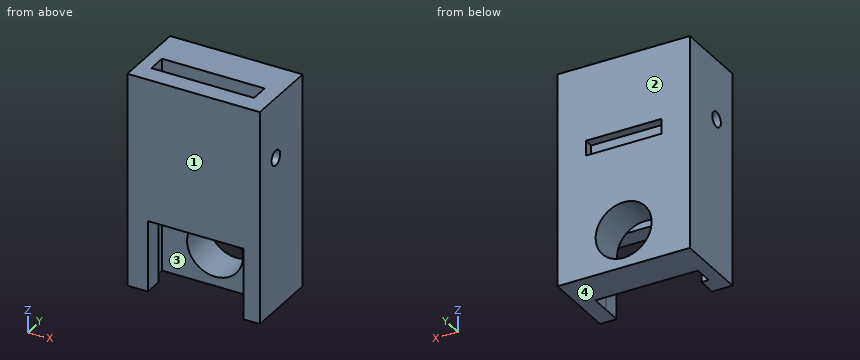
```python
from build123d import *

# Parameters (mm, degrees)
SKETCH1_W           = 71
SKETCH1_H           = 64.24
BOSS_EXTRUDE1_DEPTH = 40
SKETCH2_R           = 4
CUT_EXTRUDE2_DEPTH  = 10
SKETCH5_W           = 71
SKETCH5_H           = 40
BOSS_EXTRUDE2_DEPTH = 50
SKETCH6_R           = 15
CUT_EXTRUDE3_DEPTH  = 98.999716326
SKETCH8_W           = 40.5
SKETCH8_H           = 8
CUT_EXTRUDE5_DEPTH  = 5
CUT_EXTRUDE6_START  = -10
SKETCH9_R           = 4
CUT_EXTRUDE6_DEPTH  = 10
SKETCH10_W          = 55
SKETCH10_H          = 10
CUT_EXTRUDE7_DEPTH  = 127.138921828
SKETCH11_W          = 51.11
SKETCH11_H          = 38
CUT_EXTRUDE8_DEPTH  = 10


with BuildPart() as part:
    # Sketch1 → Boss-Extrude1 (new body)
    with BuildSketch(Plane(origin=(0, 0, 0), x_dir=(1, 0, 0), z_dir=(0, 1, 0))):
        Rectangle(SKETCH1_W, SKETCH1_H)
    extrude(amount=BOSS_EXTRUDE1_DEPTH)

    # Sketch2 → Cut-Extrude2 (cut)
    with BuildSketch(Plane.ZY.offset(35.5)):
        with Locations((-0.12, 15)):
            Circle(SKETCH2_R)
    extrude(amount=-CUT_EXTRUDE2_DEPTH, mode=Mode.SUBTRACT)

    # Sketch5 → Boss-Extrude2 (add)
    with BuildSketch(Plane(origin=(0, 0, -32.12), x_dir=(-1, 0, 0), z_dir=(0, 0, -1))):
        with Locations((0, 20)):
            Rectangle(SKETCH5_W, SKETCH5_H)
    extrude(amount=BOSS_EXTRUDE2_DEPTH)

    # Sketch6 → Cut-Extrude3 (cut, through all)
    with BuildSketch(Plane(origin=(0, 40, 0), x_dir=(1, 0, 0), z_dir=(0, 1, 0))):
        with Locations(Location((0, 62.12, 0), (0, 0, 270))):
            Circle(SKETCH6_R)
    extrude(amount=-CUT_EXTRUDE3_DEPTH, mode=Mode.SUBTRACT)

    # Sketch8 → Cut-Extrude5 (cut)
    with BuildSketch(Plane(origin=(0, 40, 0), x_dir=(1, 0, 0), z_dir=(0, 1, 0))):
        with Locations((0, 12.13)):
            Rectangle(SKETCH8_W, SKETCH8_H)
    extrude(amount=-CUT_EXTRUDE5_DEPTH, mode=Mode.SUBTRACT)

    # Sketch9 → Cut-Extrude6 (cut)
    with BuildSketch(Plane(origin=(35.5, 0, 0), x_dir=(0, 0, -1), z_dir=(1, 0, 0)).offset(CUT_EXTRUDE6_START)):
        with Locations(Location((0.12, 15, 0), (0, 0, 180))):
            Circle(SKETCH9_R)
    extrude(amount=CUT_EXTRUDE6_DEPTH, mode=Mode.SUBTRACT)

    # Sketch10 → Cut-Extrude7 (cut, through all)
    with BuildSketch(Plane.XY.offset(32.12)):
        with Locations((-0.890825636, 15)):
            Rectangle(SKETCH10_W, SKETCH10_H)
    extrude(amount=-CUT_EXTRUDE7_DEPTH, mode=Mode.SUBTRACT)

    # Sketch11 → Cut-Extrude8 (cut)
    with BuildSketch(Plane(origin=(0, 0, 0), x_dir=(-1, 0, 0), z_dir=(0, -1, 0))):
        with Locations((-1.055, 63.12)):
            Rectangle(SKETCH11_W, SKETCH11_H)
    extrude(amount=-CUT_EXTRUDE8_DEPTH, mode=Mode.SUBTRACT)


solid = part.part
```
Work out the finished part from the listing and answer in its coordinate system (mm). Face numbers are marked on the shaded views. Round coordinates to 2 decimals unless told otherwise and drop trailing zeros. Order: outer loops, then holes, each group sorted by start corner. A loop starts at its lowest first (then second) coordinate and runs counter-clockwise, first axis right, second up.
Q1. A cutting plane is placed at C-C, the plane z = -0.12. Determine the outline of the cut face in (x, y).
Solution:
outline: (-35.5, 0) - (35.5, 0) - (35.5, 11) - (26.61, 11) - (26.61, 10) - (-28.39, 10) - (-28.39, 11) - (-35.5, 11) - close; (-35.5, 19) - (-28.39, 19) - (-28.39, 20) - (26.61, 20) - (26.61, 19) - (35.5, 19) - (35.5, 40) - (-35.5, 40) - close
Q2. Given pin 1 Ø8 at (x, y) = (10.5, 5) entering from -Z; pin 2 Ø6.5 at (y, z) = (15, -0.12) entering from +X; pin 3 Ø4 at (x, z) = (9.5, -13.5) entering from +Y; pin 4 Ø1 at (x, z) = (14.5, -65.5) entering from -Y, each flat-ended and moving along its own axis, determine where each tip first touches the part or whether it passes through.
Solution:
pin 1: stops at z = -44.12
pin 2: passes through
pin 3: stops at y = 35
pin 4: stops at y = 20
Q3. Find the intervals of material crossed by line 1 along X through (y, z) = (30.25, -62.12); line 2 along Z through (x, y) = (29.5, 15); line 3 along Y through (x, z) = (33, -0.12), in increasing order.
Solution:
line 1: x = -35.5 to -15, 15 to 35.5
line 2: z = -82.12 to -4.12, 3.88 to 32.12
line 3: y = 0 to 11, 19 to 40
Q4. A cutting plane is placed at A-A, the plane x = 22. Determine the outline of the cut face in (y, z), then the cut area to 3 significant figures.
Solution:
outline: (0, -44.12) - (10, -44.12) - (10, 32.12) - (0, 32.12) - close; (20, -82.12) - (40, -82.12) - (40, 32.12) - (20, 32.12) - close
area: 3,050 mm2
Q5. A cutting plane is placed at D-D, the plane x = 0. Determine the outline of the cut face in (y, z).
Solution:
outline: (0, -44.12) - (10, -44.12) - (10, 32.12) - (0, 32.12) - close; (20, -82.12) - (40, -82.12) - (40, -77.12) - (20, -77.12) - close; (20, -47.12) - (40, -47.12) - (40, -16.13) - (35, -16.13) - (35, -8.13) - (40, -8.13) - (40, 32.12) - (20, 32.12) - close
Q6. A cutting plane is placed at B-B, the plane y = 15. Determine the outline of the cut face in (x, z).
Solution:
outline: (-35.5, -82.12) - (-28.39, -82.12) - (-28.39, -4.12) - (-35.5, -4.12) - close; (-35.5, 3.88) - (-28.39, 3.88) - (-28.39, 32.12) - (-35.5, 32.12) - close; (26.61, -82.12) - (35.5, -82.12) - (35.5, -4.12) - (26.61, -4.12) - close; (26.61, 3.88) - (35.5, 3.88) - (35.5, 32.12) - (26.61, 32.12) - close
Q7. The mould has two halves that part along Y. Classify the marked faces 1, 2, 3 and 4: pulls with the +Y half, pulls with the -Y half, needs draft (parallel to the pull), parting line crosses it, or undercut.
Solution:
face 1: pulls with the -Y half
face 2: pulls with the +Y half
face 3: undercut
face 4: needs draft
